Here's how the part is built. I have some questions about the finished solid (model axes, mm). A direction names the side the tool comes from. Give positions to 0.01 mm unless a question says otherwise; leave off trailing zeros. Loops run counter-clockwise (first coordinate to the right, second up) from the corner with the lowest first, then second, coordinate; pieces in that order, holes last. Notation, with made-up numbers: (44.25, 54) - (59.25, 54) arc R20 cw to (59.25, 80) - close; hole circle Ø9 at (42, -12). An arc over 180 degrees is marked (long way). Use a Markdown table: item, result.
from build123d import *

# Parameters (mm, degrees)
SKETCH1_W                      = 762
SKETCH1_H                      = 76.2
BASE_FLANGE1_DEPTH             = 0.75946
CUT_EXTRUDE1_DEPTH             = 10
SKETCH7_R                      = 2.8194
CUT_EXTRUDE2_DEPTH             = 10
EDGE_FLANGE1_STRIP_W           = 4.51104
EDGE_FLANGE1_STRIP_H           = 0.75946
EDGE_FLANGE1_STRIP_CUT_DEPTH   = 762
EDGE_FLANGE1_STRIP_2_W         = 4.51104
EDGE_FLANGE1_STRIP_2_H         = 0.75946
EDGE_FLANGE1_STRIP_CUT_2_DEPTH = 762
EDGE_FLANGE1_DEPTH             = 762
EDGE_FLANGE1_BEND_DEPTH        = 762
CUT_EXTRUDE4_DEPTH             = 393.47101598
CUT_EXTRUDE4_DEPTH_BACK        = 393.47101598
SKETCH42_R                     = 2.8194
EDGE_FLANGE2_STRIP_W           = 4.51104
EDGE_FLANGE2_STRIP_H           = 0.75946
EDGE_FLANGE2_STRIP_CUT_DEPTH   = 762
EDGE_FLANGE2_STRIP_2_W         = 4.51104
EDGE_FLANGE2_STRIP_2_H         = 0.75946
EDGE_FLANGE2_STRIP_CUT_2_DEPTH = 762
EDGE_FLANGE2_DEPTH             = 762
EDGE_FLANGE2_BEND_DEPTH        = 762
CUT_EXTRUDE5_REACH             = 388.993
SKETCH49_R                     = 1.651
CUT_EXTRUDE6_DEPTH             = 393.578884814
CUT_EXTRUDE6_DEPTH_BACK        = 393.578884814
SKETCH50_R                     = 2.8194


# Sheet-metal steps are written as plain solids
with BuildPart() as part:
    # Sketch1 → Base-Flange1 (new body)
    with BuildSketch(Plane(origin=(0, 0, 0), x_dir=(1, 0, 0), z_dir=(0, 1, 0))):
        Rectangle(SKETCH1_W, SKETCH1_H)
    extrude(amount=-BASE_FLANGE1_DEPTH)

    # Sketch6 → Cut-Extrude1 (cut)
    with BuildSketch(Plane(origin=(0, 0, 0), x_dir=(1, 0, 0), z_dir=(0, 1, 0))):
        Polygon((53.7835, 19.05), (64.8335, 19.05), (64.8335, -19.05), (53.7835, -19.05), (30.1625, -19.05), (30.1625, 19.05), align=None)
    extrude(amount=-CUT_EXTRUDE1_DEPTH, mode=Mode.SUBTRACT)

    # Sketch7 → Cut-Extrude2 (cut)
    with BuildSketch(Plane(origin=(0, 0, 0), x_dir=(1, 0, 0), z_dir=(0, 1, 0))):
        with Locations(Location((20.0625, 0, 0), (0, 0, 270))):
            Circle(SKETCH7_R)
        with Locations(Location((74.9335, 0, 0), (0, 0, 270))):
            Circle(SKETCH7_R)
    extrude(amount=-CUT_EXTRUDE2_DEPTH, mode=Mode.SUBTRACT)

    # Edge-Flange1 strip (across the edge) → Edge-Flange1 strip cut (cut)
    with BuildSketch(Plane(origin=(-381, -0.75946, -38.1), x_dir=(0, 0, 1), z_dir=(1, 0, 0))):
        with Locations((-0.75946, -0.37973)):
            Rectangle(EDGE_FLANGE1_STRIP_W, EDGE_FLANGE1_STRIP_H)
    extrude(amount=EDGE_FLANGE1_STRIP_CUT_DEPTH, mode=Mode.SUBTRACT)

    # Edge-Flange1 strip 2 (across the edge) → Edge-Flange1 strip cut 2 (cut)
    with BuildSketch(Plane(origin=(381, -0.75946, 38.1), x_dir=(0, 0, -1), z_dir=(-1, 0, 0))):
        with Locations((-0.75946, -0.37973)):
            Rectangle(EDGE_FLANGE1_STRIP_2_W, EDGE_FLANGE1_STRIP_2_H)
    extrude(amount=EDGE_FLANGE1_STRIP_CUT_2_DEPTH, mode=Mode.SUBTRACT)

    # Edge-Flange1 section (across the edge) → Edge-Flange1 (add)
    with BuildSketch(Plane(origin=(-381, -0.75946, -38.1), x_dir=(0, 0, 1), z_dir=(1, 0, 0))):
        with BuildLine():
            Line((0, 0.7366), (0, 54.61254))
            Line((0, 54.61254), (0.75946, 54.61254))
            Line((0.75946, 54.61254), (0.75946, 0.7366))
            ThreePointArc((0.75946, 0.7366), (0.975205145, 0.215745145), (1.49606, 0))
            Line((1.49606, 0), (1.49606, -0.75946))
            ThreePointArc((1.49606, -0.75946), (0.438185829, -0.321274171), (0, 0.7366))
        make_face()
    extrude(amount=EDGE_FLANGE1_DEPTH)

    # Edge-Flange1 section 2 (across the edge) → Edge-Flange1 bend (add)
    with BuildSketch(Plane(origin=(381, -0.75946, 38.1), x_dir=(0, 0, -1), z_dir=(-1, 0, 0))):
        with BuildLine():
            Line((0, 0.7366), (0, 54.61254))
            Line((0, 54.61254), (0.75946, 54.61254))
            Line((0.75946, 54.61254), (0.75946, 0.7366))
            ThreePointArc((0.75946, 0.7366), (0.975205145, 0.215745145), (1.49606, 0))
            Line((1.49606, 0), (1.49606, -0.75946))
            ThreePointArc((1.49606, -0.75946), (0.438185829, -0.321274171), (0, 0.7366))
        make_face()
    extrude(amount=EDGE_FLANGE1_BEND_DEPTH)

    # Sketch42 → Cut-Extrude4 (cut, two sides: drawn at the far end of the back side and taken through both)
    with BuildSketch(Plane(origin=(0, 0, -38.1), x_dir=(-1, 0, 0), z_dir=(0, 0, -1)).offset(-CUT_EXTRUDE4_DEPTH_BACK)):
        with Locations(Location((-359.41, -13.45946, 0), (0, 0, 90))):
            Circle(SKETCH42_R)
        with Locations(Location((-359.41, -42.164, 0), (0, 0, 90))):
            Circle(SKETCH42_R)
    extrude(amount=CUT_EXTRUDE4_DEPTH + CUT_EXTRUDE4_DEPTH_BACK, mode=Mode.SUBTRACT)

    # Edge-Flange2 strip (across the edge) → Edge-Flange2 strip cut (cut)
    with BuildSketch(Plane(origin=(-381, -55.372, -37.34054), x_dir=(0, 1, 0), z_dir=(1, 0, 0))):
        with Locations((-1.51892, -0.37973)):
            Rectangle(EDGE_FLANGE2_STRIP_W, EDGE_FLANGE2_STRIP_H)
    extrude(amount=EDGE_FLANGE2_STRIP_CUT_DEPTH, mode=Mode.SUBTRACT)

    # Edge-Flange2 strip 2 (across the edge) → Edge-Flange2 strip cut 2 (cut)
    with BuildSketch(Plane(origin=(381, -55.372, 37.34054), x_dir=(0, 1, 0), z_dir=(-1, 0, 0))):
        with Locations((-1.51892, -0.37973)):
            Rectangle(EDGE_FLANGE2_STRIP_2_W, EDGE_FLANGE2_STRIP_2_H)
    extrude(amount=EDGE_FLANGE2_STRIP_CUT_2_DEPTH, mode=Mode.SUBTRACT)

    # Edge-Flange2 section (across the edge) → Edge-Flange2 (add)
    with BuildSketch(Plane(origin=(-381, -55.372, -37.34054), x_dir=(0, 1, 0), z_dir=(1, 0, 0))):
        with BuildLine():
            Line((-0.75946, 0.7366), (-0.75946, 9.40054))
            Line((-0.75946, 9.40054), (0, 9.40054))
            Line((0, 9.40054), (0, 0.7366))
            ThreePointArc((0, 0.7366), (0.215745145, 0.215745145), (0.7366, 0))
            Line((0.7366, 0), (0.7366, -0.75946))
            ThreePointArc((0.7366, -0.75946), (-0.321274171, -0.321274171), (-0.75946, 0.7366))
        make_face()
    extrude(amount=EDGE_FLANGE2_DEPTH)

    # Edge-Flange2 section 2 (across the edge) → Edge-Flange2 bend (add)
    with BuildSketch(Plane(origin=(381, -55.372, 37.34054), x_dir=(0, 1, 0), z_dir=(-1, 0, 0))):
        with BuildLine():
            Line((-0.75946, 0.7366), (-0.75946, 9.40054))
            Line((-0.75946, 9.40054), (0, 9.40054))
            Line((0, 9.40054), (0, 0.7366))
            ThreePointArc((0, 0.7366), (0.215745145, 0.215745145), (0.7366, 0))
            Line((0.7366, 0), (0.7366, -0.75946))
            ThreePointArc((0.7366, -0.75946), (-0.321274171, -0.321274171), (-0.75946, 0.7366))
        make_face()
    extrude(amount=EDGE_FLANGE2_BEND_DEPTH)

    # Sketch49 → Cut-Extrude5 (cut, up to next)
    with BuildSketch(Plane.XZ.offset(56.13146), mode=Mode.PRIVATE) as cut_extrude5_sk1:
        with Locations(Location((254, -32.79394, 0), (0, 0, 270))):
            Circle(SKETCH49_R)
    cut_extrude5_tool1 = extrude(cut_extrude5_sk1.sketch, amount=-CUT_EXTRUDE5_REACH, mode=Mode.PRIVATE) & part.part
    # Sketch49 → Cut-Extrude5 (cut, up to next)
    with BuildSketch(Plane.XZ.offset(56.13146), mode=Mode.PRIVATE) as cut_extrude5_sk2:
        with Locations(Location((254, 32.79394, 0), (0, 0, 270))):
            Circle(SKETCH49_R)
    cut_extrude5_tool2 = extrude(cut_extrude5_sk2.sketch, amount=-CUT_EXTRUDE5_REACH, mode=Mode.PRIVATE) & part.part
    # Sketch49 → Cut-Extrude5 (cut, up to next)
    with BuildSketch(Plane.XZ.offset(56.13146), mode=Mode.PRIVATE) as cut_extrude5_sk3:
        with Locations(Location((0, 32.79394, 0), (0, 0, 270))):
            Circle(SKETCH49_R)
    cut_extrude5_tool3 = extrude(cut_extrude5_sk3.sketch, amount=-CUT_EXTRUDE5_REACH, mode=Mode.PRIVATE) & part.part
    # Sketch49 → Cut-Extrude5 (cut, up to next)
    with BuildSketch(Plane.XZ.offset(56.13146), mode=Mode.PRIVATE) as cut_extrude5_sk4:
        with Locations(Location((0, -32.79394, 0), (0, 0, 270))):
            Circle(SKETCH49_R)
    cut_extrude5_tool4 = extrude(cut_extrude5_sk4.sketch, amount=-CUT_EXTRUDE5_REACH, mode=Mode.PRIVATE) & part.part
    # Sketch49 → Cut-Extrude5 (cut, up to next)
    with BuildSketch(Plane.XZ.offset(56.13146), mode=Mode.PRIVATE) as cut_extrude5_sk5:
        with Locations(Location((-304.8, -32.79394, 0), (0, 0, 270))):
            Circle(SKETCH49_R)
    cut_extrude5_tool5 = extrude(cut_extrude5_sk5.sketch, amount=-CUT_EXTRUDE5_REACH, mode=Mode.PRIVATE) & part.part
    # Sketch49 → Cut-Extrude5 (cut, up to next)
    with BuildSketch(Plane.XZ.offset(56.13146), mode=Mode.PRIVATE) as cut_extrude5_sk6:
        with Locations(Location((-304.8, 32.79394, 0), (0, 0, 270))):
            Circle(SKETCH49_R)
    cut_extrude5_tool6 = extrude(cut_extrude5_sk6.sketch, amount=-CUT_EXTRUDE5_REACH, mode=Mode.PRIVATE) & part.part
    # Sketch49 → Cut-Extrude5 (cut, up to next)
    with BuildSketch(Plane.XZ.offset(56.13146), mode=Mode.PRIVATE) as cut_extrude5_sk7:
        with Locations(Location((-355.6, 32.79394, 0), (0, 0, 270))):
            Circle(SKETCH49_R)
    cut_extrude5_tool7 = extrude(cut_extrude5_sk7.sketch, amount=-CUT_EXTRUDE5_REACH, mode=Mode.PRIVATE) & part.part
    # Sketch49 → Cut-Extrude5 (cut, up to next)
    with BuildSketch(Plane.XZ.offset(56.13146), mode=Mode.PRIVATE) as cut_extrude5_sk8:
        with Locations(Location((-355.6, -32.79394, 0), (0, 0, 270))):
            Circle(SKETCH49_R)
    cut_extrude5_tool8 = extrude(cut_extrude5_sk8.sketch, amount=-CUT_EXTRUDE5_REACH, mode=Mode.PRIVATE) & part.part
    # Sketch49 → Cut-Extrude5 (cut, up to next)
    with BuildSketch(Plane.XZ.offset(56.13146), mode=Mode.PRIVATE) as cut_extrude5_sk9:
        with Locations(Location((355.6, -32.79394, 0), (0, 0, 270))):
            Circle(SKETCH49_R)
    cut_extrude5_tool9 = extrude(cut_extrude5_sk9.sketch, amount=-CUT_EXTRUDE5_REACH, mode=Mode.PRIVATE) & part.part
    # Sketch49 → Cut-Extrude5 (cut, up to next)
    with BuildSketch(Plane.XZ.offset(56.13146), mode=Mode.PRIVATE) as cut_extrude5_sk10:
        with Locations(Location((355.6, 32.79394, 0), (0, 0, 270))):
            Circle(SKETCH49_R)
    cut_extrude5_tool10 = extrude(cut_extrude5_sk10.sketch, amount=-CUT_EXTRUDE5_REACH, mode=Mode.PRIVATE) & part.part
    # Sketch49 → Cut-Extrude5 (cut, up to next)
    with BuildSketch(Plane.XZ.offset(56.13146), mode=Mode.PRIVATE) as cut_extrude5_sk11:
        with Locations(Location((152.4, 32.79394, 0), (0, 0, 270))):
            Circle(SKETCH49_R)
    cut_extrude5_tool11 = extrude(cut_extrude5_sk11.sketch, amount=-CUT_EXTRUDE5_REACH, mode=Mode.PRIVATE) & part.part
    # Sketch49 → Cut-Extrude5 (cut, up to next)
    with BuildSketch(Plane.XZ.offset(56.13146), mode=Mode.PRIVATE) as cut_extrude5_sk12:
        with Locations(Location((152.4, -32.79394, 0), (0, 0, 270))):
            Circle(SKETCH49_R)
    cut_extrude5_tool12 = extrude(cut_extrude5_sk12.sketch, amount=-CUT_EXTRUDE5_REACH, mode=Mode.PRIVATE) & part.part
    # Sketch49 → Cut-Extrude5 (cut, up to next)
    with BuildSketch(Plane.XZ.offset(56.13146), mode=Mode.PRIVATE) as cut_extrude5_sk13:
        with Locations(Location((-152.4, 32.79394, 0), (0, 0, 270))):
            Circle(SKETCH49_R)
    cut_extrude5_tool13 = extrude(cut_extrude5_sk13.sketch, amount=-CUT_EXTRUDE5_REACH, mode=Mode.PRIVATE) & part.part
    # Sketch49 → Cut-Extrude5 (cut, up to next)
    with BuildSketch(Plane.XZ.offset(56.13146), mode=Mode.PRIVATE) as cut_extrude5_sk14:
        with Locations(Location((-152.4, -32.79394, 0), (0, 0, 270))):
            Circle(SKETCH49_R)
    cut_extrude5_tool14 = extrude(cut_extrude5_sk14.sketch, amount=-CUT_EXTRUDE5_REACH, mode=Mode.PRIVATE) & part.part
    add(cut_extrude5_tool1.solids().sort_by_distance((254, -56.13146, -32.79394))[0], mode=Mode.SUBTRACT)
    add(cut_extrude5_tool2.solids().sort_by_distance((254, -56.13146, 32.79394))[0], mode=Mode.SUBTRACT)
    add(cut_extrude5_tool3.solids().sort_by_distance((0, -56.13146, 32.79394))[0], mode=Mode.SUBTRACT)
    add(cut_extrude5_tool4.solids().sort_by_distance((0, -56.13146, -32.79394))[0], mode=Mode.SUBTRACT)
    add(cut_extrude5_tool5.solids().sort_by_distance((-304.8, -56.13146, -32.79394))[0], mode=Mode.SUBTRACT)
    add(cut_extrude5_tool6.solids().sort_by_distance((-304.8, -56.13146, 32.79394))[0], mode=Mode.SUBTRACT)
    add(cut_extrude5_tool7.solids().sort_by_distance((-355.6, -56.13146, 32.79394))[0], mode=Mode.SUBTRACT)
    add(cut_extrude5_tool8.solids().sort_by_distance((-355.6, -56.13146, -32.79394))[0], mode=Mode.SUBTRACT)
    add(cut_extrude5_tool9.solids().sort_by_distance((355.6, -56.13146, -32.79394))[0], mode=Mode.SUBTRACT)
    add(cut_extrude5_tool10.solids().sort_by_distance((355.6, -56.13146, 32.79394))[0], mode=Mode.SUBTRACT)
    add(cut_extrude5_tool11.solids().sort_by_distance((152.4, -56.13146, 32.79394))[0], mode=Mode.SUBTRACT)
    add(cut_extrude5_tool12.solids().sort_by_distance((152.4, -56.13146, -32.79394))[0], mode=Mode.SUBTRACT)
    add(cut_extrude5_tool13.solids().sort_by_distance((-152.4, -56.13146, 32.79394))[0], mode=Mode.SUBTRACT)
    add(cut_extrude5_tool14.solids().sort_by_distance((-152.4, -56.13146, -32.79394))[0], mode=Mode.SUBTRACT)

    # Sketch50 → Cut-Extrude6 (cut, two sides: drawn at the far end of the back side and taken through both)
    with BuildSketch(Plane.XY.offset(38.1).offset(-CUT_EXTRUDE6_DEPTH_BACK)):
        with Locations((-372.618, -29.21)):
            Circle(SKETCH50_R)
    extrude(amount=CUT_EXTRUDE6_DEPTH + CUT_EXTRUDE6_DEPTH_BACK, mode=Mode.SUBTRACT)


solid = part.part
(1) On a 3-axis mill with a long thin cutter (end or side, diameter ignored), from which of +Z, -Z, +X, -X, +Y, -Y can I reach the whole of each face in a straight line? I mean faces 5 (the face through (-5, -28, -37.341)), 6 (the face through (5, -28, 38.1)). Say none if no direction works.
A:
| item | result |
|---|---|
| face 5 | +X, -X |
| face 6 | +Z, +X, -X, +Y, -Y |
(2) Will these pins go through, and if not, where does the flat tip stop? pin 1 (2.5 mm diameter, centred on x = 355.6, z = 32.79, fed in from -Y); pin 2 (4 mm diameter, centred on x = 355.6, z = -32.79, fed in from +Y); pin 3 (5 mm diameter, centred on y = -5.5, z = -3.5, fed in from -X).
A:
| item | result |
|---|---|
| pin 1 | y = -0.76 |
| pin 2 | y = 0 |
| pin 3 | through |
(3) Suppose I cut it at B-B on x = -141. Write out the boundary of the cut face in (y, z).
A:
| item | result |
|---|---|
| outline | (-56.13, -36.6) arc R1.5 ccw to (-54.64, -38.1) - (-1.5, -38.1) arc R1.5 ccw to (0, -36.6) - (0, 36.6) arc R1.5 ccw to (-1.5, 38.1) - (-54.64, 38.1) arc R1.5 ccw to (-56.13, 36.6) - (-56.13, 27.94) - (-55.37, 27.94) - (-55.37, 36.6) arc R0.74 cw to (-54.64, 37.34) - (-1.5, 37.34) arc R0.74 cw to (-0.76, 36.6) - (-0.76, -36.6) arc R0.74 cw to (-1.5, -37.34) - (-54.64, -37.34) arc R0.74 cw to (-55.37, -36.6) - (-55.37, -27.94) - (-56.13, -27.94) - close |
(4) Suppose I cut it at A-A on x = 48. Write out the boundary of the cut face in (y, z), plus the area to 3 significant figures.
A:
| item | result |
|---|---|
| outline | (-56.13, -36.6) arc R1.5 ccw to (-54.64, -38.1) - (-1.5, -38.1) arc R1.5 ccw to (0, -36.6) - (0, -19.05) - (-0.76, -19.05) - (-0.76, -36.6) arc R0.74 cw to (-1.5, -37.34) - (-54.64, -37.34) arc R0.74 cw to (-55.37, -36.6) - (-55.37, -27.94) - (-56.13, -27.94) - close; (-56.13, 27.94) - (-55.37, 27.94) - (-55.37, 36.6) arc R0.74 cw to (-54.64, 37.34) - (-1.5, 37.34) arc R0.74 cw to (-0.76, 36.6) - (-0.76, 19.05) - (0, 19.05) - (0, 36.6) arc R1.5 ccw to (-1.5, 38.1) - (-54.64, 38.1) arc R1.5 ccw to (-56.13, 36.6) - close |
| area | 126 mm2 |
(5) If I drill on line 1 (Z direction, x = -152.4, y = -55.9); line 2 (Z direction, x = -304, y = -55); line 3 (Z direction, x = -152.4, y = -55.55), over which ranges is the centre line in solid material (lowest first)?
A:
| item | result |
|---|---|
| line 1 | -37.4 to -34.44, -31.14 to -27.94, 27.94 to 31.14, 34.44 to 37.4 |
| line 2 | -38.05 to -37.24, 37.24 to 38.05 |
| line 3 | -37.79 to -34.44, -31.14 to -27.94, 27.94 to 31.14, 34.44 to 37.79 |
(6) We'd pull the mould along Z, two halves only. Please class faces 1 (the face through (-5, 0, -1)), 2 (the face through (-5, -28, -38.1)), 3 (the face through (-5, -0.759, -1)), 4 (the face through (5, -28, 37.341)): pulls with the +Z half, pulls with the -Z half, needs draft (parallel to the pull), parting line crosses it, or undercut.
A:
| item | result |
|---|---|
| face 1 | needs draft |
| face 2 | pulls with the -Z half |
| face 3 | undercut |
| face 4 | undercut |
